```python
from build123d import *

# Parameters (mm, degrees)
SKETCH1_R         = 25.4
EXTRUDE1_DEPTH    = 1.5875
EXTRUDE2_START    = 1.5875
SKETCH1_3_R       = 53.975
EXTRUDE2_DEPTH    = 12.7
EXTRUDE3_START    = 14.2875
SKETCH1_4_R       = 16.764
EXTRUDE3_DEPTH    = 41.275
EXTRUDE4_START    = 1.5875
SKETCH1_5_R       = 7.9375
EXTRUDE4_DEPTH    = 12.7
CIRPATTERN1_COUNT = 4
EXTRUDE5_REACH    = 96.413
SKETCH3_R         = 13.3223


with BuildPart() as part:
    # Sketch1 → Extrude1 (new body)
    with BuildSketch(Plane.XY):
        Circle(SKETCH1_R)
    extrude(amount=EXTRUDE1_DEPTH)

    # Sketch1<3> → Extrude2 (add)
    with BuildSketch(Plane.XY.offset(EXTRUDE2_START)):
        Circle(SKETCH1_3_R)
    extrude(amount=EXTRUDE2_DEPTH)

    # Sketch1<4> → Extrude3 (add)
    with BuildSketch(Plane.XY.offset(EXTRUDE3_START)):
        Circle(SKETCH1_4_R)
    extrude(amount=EXTRUDE3_DEPTH)

    # Sketch4 → Revolve1 (revolve)
    with BuildSketch(Plane(origin=(0, 0, 0), x_dir=(0, 0, -1), z_dir=(1, 0, 0)), mode=Mode.PRIVATE) as revolve1_sk:
        Polygon((-42.8625, 16.764), (-14.2875, 24.60625), (-14.2875, 16.764), align=None)
    revolve(revolve1_sk.sketch.rotate(Axis((0, 0, -2.619375), (0, 0, 1)), 90), axis=Axis((0, 0, -2.619375), (0, 0, 1)))

    # Sketch1<5> → Extrude4 (cut)
    with BuildSketch(Plane.XY.offset(EXTRUDE4_START)):
        with Locations((0, 39.6875)):
            Circle(SKETCH1_5_R)
    extrude4 = extrude(amount=EXTRUDE4_DEPTH, mode=Mode.SUBTRACT)

    # CirPattern1: Extrude4 ×4 about axis
    cirpattern1_axis = Axis((0, 0, 0), (0, 0, 1))
    for i in range(1, CIRPATTERN1_COUNT):
        add(extrude4.rotate(cirpattern1_axis, i * 360 / CIRPATTERN1_COUNT), mode=Mode.SUBTRACT)

    # Sketch3 → Extrude5 (cut, up to next)
    with BuildSketch(Plane(origin=(0, 0, 55.5625), x_dir=(-1, 0, 0), z_dir=(0, 0, -1)), mode=Mode.PRIVATE) as extrude5_sk1:
        with Locations(Location((0, 0, 0), (0, 0, 180))):
            Circle(SKETCH3_R)
    extrude5_tool1 = extrude(extrude5_sk1.sketch, amount=EXTRUDE5_REACH, mode=Mode.PRIVATE) & part.part
    add(extrude5_tool1.solids().sort_by_distance((0, 0, 55.5625))[0], mode=Mode.SUBTRACT)

    # Sketch5 → Cut-Revolve1 (revolve, cut)
    with BuildSketch(Plane(origin=(0, 0, 0), x_dir=(0, 0, -1), z_dir=(1, 0, 0)), mode=Mode.PRIVATE) as cut_revolve1_sk:
        Polygon((-55.5625, 16.764), (-53.530656502, 16.764), (-55.5625, 14.11605), align=None)
    revolve(cut_revolve1_sk.sketch.rotate(Axis((0, 0, -2.619375), (0, 0, 1)), 90), axis=Axis((0, 0, -2.619375), (0, 0, 1)), mode=Mode.SUBTRACT)


solid = part.part
```
Part model, mm, in its own coordinate system. A direction names the side the tool comes from. Give positions to 0.01 mm unless a question says otherwise; leave off trailing zeros. Write each loop counter-clockwise with the first axis right and the second up, starting at its lowest first coordinate (ties: lowest second). Pieces come first, ordered by that corner, then holes. Notation, with made-up numbers: (3.25, 83.5) -> (19.25, 83.5) arc R24 ccw to (19.25, 97.5) -> close; hole circle Ø5 at (40.5, 52). An arc over 180 degrees is marked (long way). Put each result on its own line as item: value. Start each with the question number.
Item 1: Cut at A-A (y = 0). State how many separate pieces and enclosed holes the cut face has, then the cut area to 3 significant figures.
Item 2: Wall check: L1, parallel to Y at x = 0, z = 4.5 (3 decimals); L2, parallel to X at y = 4, z = 6; L3, parallel to Z at x = -32, y = -41. Give the ranges that are in metal, low to high. Write a range as [from, to].
Item 3: Pull direction Y, two halves, no side cores. Call faces 4 (the face through (11.304, 8.668, 55.464)), 5 (the face through (12.5, -5.2, 55.562)), 6 (the face through (31.94, 1.72, 7.85)): pulls with the +Y half, pulls with the -Y half, needs draft (parallel to the pull), parting line crosses it, or undercut.
Item 4: Cut at D-D (x = 42). List the corners of the cut face in (y, z), then the cut area to 3 significant figures.
Item 5: Pin check, flat tips, straight feed: pin 1 Ø3 at (x, z) = (13, 37) entering from -Y; pin 2 Ø12 at (x, y) = (-30.5, 37) entering from -Z; pin 3 Ø21.5 at (x, y) = (0, 0) entering from -Z; pin 4 Ø8 at (y, z) = (-17, 43) entering from -X. Stop position of each tip, or through.
Item 6: Which spindle directions (+Z, -Z, +X, -X, +Y, -Y) get a long thin tool onto all of the face, cutting with end or side? Do faces 1 (the face through (16, 5, 48)), 2 (the face through (1.72, -31.94, 7.85)), 3 (the face through (-5.506, -24.796, 0.783)). Say none if no direction does.
Answer list:
1. separate pieces: 4
1. enclosed holes: 0
1. area: 1,170 mm2
2. L1: y = [-53.975, -47.625], [-31.75, -13.322], [13.322, 31.75], [47.625, 53.975]
2. L2: x = [-53.83, -46.54], [-32.83, -12.71], [12.71, 32.83], [46.54, 53.83]
2. L3: z = [1.59, 14.29]
3. face 4: parting line crosses it
3. face 5: needs draft
3. face 6: undercut
4. outline: (-33.9, 1.59) -> (-7.59, 1.59) -> (-7.59, 14.29) -> (-33.9, 14.29) -> close; (7.59, 1.59) -> (33.9, 1.59) -> (33.9, 14.29) -> (7.59, 14.29) -> close
4. area: 668 mm2
5. pin 1: stops at y = -14.44
5. pin 2: stops at z = 1.59
5. pin 3: passes through
5. pin 4: stops at x = -10.82
6. face 1: +Z
6. face 2: +Z, -Z
6. face 3: -Z
